Check sheet for the modelled part. Datum: model origin and axes. Units: mm. Coordinates: 2 decimals unless noted, no trailing zeros. Write each loop counter-clockwise with the first axis right and the second up, starting at its lowest first coordinate (ties: lowest second). Pieces come first, ordered by that corner, then holes. Notation, with made-up numbers: M -40,41.25 L -18,41.25 A30 ccw -18,65.25 Z; hole C 64,67.25 d9. An arc over 180 degrees is marked long. Answer as CSV lines item,"result".
from build123d import *

# Parameters (mm, degrees)
F2_R          = 3.81
F2_R_2        = 1.27
F3_DEPTH      = 2.032
F3_DEPTH_BACK = 2.032


with BuildPart() as f1:
    # F0 (on Front) → F1 (revolve)
    with BuildSketch(Plane.XZ):
        with BuildLine():
            Line((0, 0), (0, -88.756312))
            ThreePointArc((0, -88.756312), (12.382447, -78.878546), (5.503333, -64.610644))
            ThreePointArc((5.503333, -64.610644), (2.879333, -62.267855), (1.905, -58.88781))
            Line((1.905, -58.88781), (1.905, 0))
            Line((1.905, 0), (0, 0))
        make_face()
    revolve(axis=Axis((0, 0, -44.378156), (0, 0, 1)))

    # F2 (on Front) → F3 (join, two sides)
    with BuildSketch(Plane.XZ) as f3_sk:
        with Locations((0, 2.379173)):
            Circle(F2_R)
        with Locations((0, 2.379173)):
            Circle(F2_R_2, mode=Mode.SUBTRACT)
    extrude(amount=F3_DEPTH)
    extrude(f3_sk.sketch, amount=-F3_DEPTH_BACK)


solid = f1.part
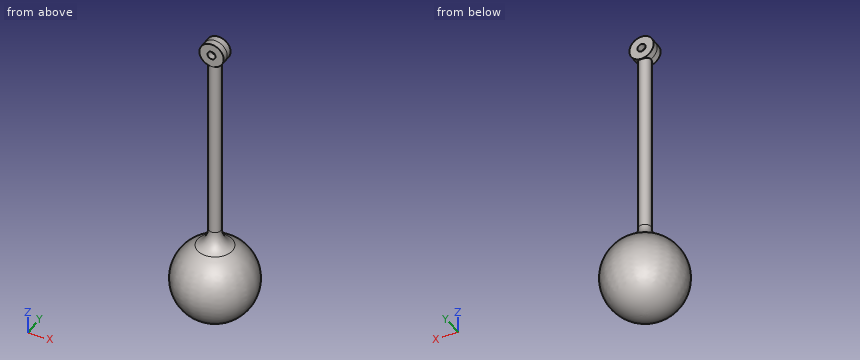
1) Section check B-B, the plane z = -60. Record the boundary of the cut face in (x, y), plus the area to 3 significant figures.
Answer key:
outline,"C 0,0 d4.01"
area,"12.6 mm2"
2) Depth check by flat-ended pin: P1, Ø3, axis at x = 0, z = 2.38, coming from the +Y side; P2, Ø6, axis at x = 4, z = -43.5, coming from the -Y side; P3, Ø3, axis at x = 3.5, z = -14, coming from the -Y side; P4, Ø1.5, axis at x = 8.5, y = 2, coming from the -Z side. Enter the tip coordinate at first touch or a pass-through.
Answer key:
P1,"stops at y = 2.03"
P2,"stops at y = -1.62"
P3,"passes through"
P4,"stops at z = -85.93"
3) Thickness scan on line 1 along X through (y, z) = (-0.25, -13); line 2 along Z through (x, y) = (0, 1.15); line 3 along Y through (x, z) = (0, -75.5). Record the ranges inside material, lowest first.
Answer key:
line 1,"x = -1.89 to 1.89"
line 2,"z = -88.7 to 1.11, 3.65 to 6.19"
line 3,"y = -12.69 to 12.69"
4) Section check A-A, the plane z = -32. Record the boundary of the cut face in (x, y) (3 decimals), plus the area to 3 significant figures.
Answer key:
outline,"C 0,0 d3.81"
area,"11.4 mm2"
